Source: CAD feature listing. Evaluate the final solid. Frame: model axes, mm. A direction names the side the tool comes from. Round coordinates to 2 decimals unless told otherwise and drop trailing zeros. Order: outer loops, then holes, each group sorted by start corner. A loop starts at its lowest first (then second) coordinate and runs counter-clockwise, first axis right, second up. Notation, with made-up numbers: (-22, -33.75) -> (2, -33.75) arc R27 cw to (2, -14.75) -> close; hole circle Ø11 at (2.25, 8). An arc over 180 degrees is marked (long way). Answer as CSV lines item,"result".
from build123d import *

# Parameters (mm, degrees)
SKETCH1_W          = 30
SKETCH1_H          = 30
EXTRUDE1_DEPTH     = 500
SKETCH2_W          = 22
SKETCH2_H          = 22
CUT_EXTRUDE1_DEPTH = 500
SKETCH3_W          = 200
SKETCH3_H          = 20
EXTRUDE2_DEPTH     = 4
SKETCH4_W          = 30
SKETCH4_H          = 200
EXTRUDE3_DEPTH     = 12
SKETCH6_W          = 30
SKETCH6_H          = 220
EXTRUDE4_DEPTH     = 3


with BuildPart() as part:
    # Sketch1 → Extrude1 (new body)
    with BuildSketch(Plane(origin=(0, 0, 0), x_dir=(1, 0, 0), z_dir=(0, 1, 0))):
        Rectangle(SKETCH1_W, SKETCH1_H)
    extrude(amount=EXTRUDE1_DEPTH)

    # Sketch2 → Cut-Extrude1 (cut)
    with BuildSketch(Plane(origin=(0, 500, 0), x_dir=(1, 0, 0), z_dir=(0, 1, 0))):
        Rectangle(SKETCH2_W, SKETCH2_H)
    extrude(amount=-CUT_EXTRUDE1_DEPTH, mode=Mode.SUBTRACT)

    # Sketch3 → Extrude2 (add)
    with BuildSketch(Plane(origin=(0, 500, 0), x_dir=(1, 0, 0), z_dir=(0, 1, 0))):
        with Locations((20, 0)):
            Rectangle(SKETCH3_W, SKETCH3_H)
    extrude(amount=EXTRUDE2_DEPTH)

    # Sketch4 → Extrude3 (add)
    with BuildSketch(Plane(origin=(15, 0, 0), x_dir=(0, 0, -1), z_dir=(1, 0, 0))):
        with Locations((0, 110)):
            Rectangle(SKETCH4_W, SKETCH4_H)
    extrude(amount=EXTRUDE3_DEPTH)

    # Sketch6 → Extrude4 (add)
    with BuildSketch(Plane(origin=(15, 0, 0), x_dir=(0, 0, -1), z_dir=(1, 0, 0))):
        with Locations((0, 371.238460257)):
            Rectangle(SKETCH6_W, SKETCH6_H)
    extrude(amount=EXTRUDE4_DEPTH)


solid = part.part
1. Pin query (flat end, axial travel): pin 1 (2.5 mm diameter, centred on x = 1.5, z = -12, fed in from +Y); pin 2 (15 mm diameter, centred on y = 405.5, z = 5.5, fed in from +X); pin 3 (1.5 mm diameter, centred on x = -52, z = 10, fed in from -Y). Return the tip coordinate at first contact, or that it passes through.
Results below:
pin 1,"y = 500"
pin 2,"x = 18"
pin 3,"y = 500"
2. Line query: L1, parallel to X at y = 82, z = 2.75; L2, parallel to X at y = 252, z = -1. Output: solid intervals per line, ascending. Write a range as [from, to].
Results below:
L1,"[-15, -11], [11, 27]"
L2,"[-15, -11], [11, 15]"
3. Reachability of faces 1 (the flat face through (15, 235, 0)), 2 (the flat face through (0, 500, 0)), 3 (the flat face through (0, 254, -11)), 4 (the flat face through (27, 111, 0)), 5 (the flat face through (-48, 500, 0)) from +Z, -Z, +X, -X, +Y, -Y: full face, straight path, thin tool, end or side. Return the list, or none.
Results below:
face 1,"+Z, -Z, +X"
face 2,"-Y"
face 3,"+Y, -Y"
face 4,"+Z, -Z, +X, -Y"
face 5,"+Z, -Z, -X, -Y"
4. Mould query, pull axis X, two halves, no side actions, for faces 6 (the flat face through (-15, 246, 0)), 7 (the flat face through (1, 246, -15)), 8 (the flat face through (11, 254, 0)). Classes: released by +X, released by -X, zero draft, split by the parting line, or undercut.
Results below:
face 6,"released by -X"
face 7,"zero draft"
face 8,"undercut"
5. Section query C-C on y = 428. Return loops of the section in (x, z), and give its area (3 significant figures).
Results below:
outline,"(-15, -15) -> (18, -15) -> (18, 15) -> (-15, 15) -> close; hole (-11, -11) -> (11, -11) -> (11, 11) -> (-11, 11) -> close"
area,"506 mm2"
6. Section query A-A on y = 51. Return loops of the section in (x, z), and give its area (3 significant figures).
Results below:
outline,"(-15, -15) -> (27, -15) -> (27, 15) -> (-15, 15) -> close; hole (-11, -11) -> (11, -11) -> (11, 11) -> (-11, 11) -> close"
area,"776 mm2"
7. Section query D-D on x = 87.5. Return loops of the section in (y, z), and give its area (3 significant figures).
Results below:
outline,"(500, -10) -> (504, -10) -> (504, 10) -> (500, 10) -> close"
area,"80.0 mm2"
8. Section query B-B on z = 4.5. Return loops of the section in (x, y).
Results below:
outline,"(-80, 500) -> (-15, 500) -> (-15, 0) -> (-11, 0) -> (-11, 500) -> (11, 500) -> (11, 0) -> (15, 0) -> (15, 10) -> (27, 10) -> (27, 210) -> (15, 210) -> (15, 261.24) -> (18, 261.24) -> (18, 481.24) -> (15, 481.24) -> (15, 500) -> (120, 500) -> (120, 504) -> (-80, 504) -> close"
